Could you check a few things on this model? Use its own coordinates, in mm. A direction names the side the tool comes from. Give positions to 0.01 mm unless a question says otherwise; leave off trailing zeros. Loops run counter-clockwise (first coordinate to the right, second up) from the corner with the lowest first, then second, coordinate; pieces in that order, holes last. Notation, with made-up numbers: (-34, 17.25) - (-3, 17.25) arc R25 cw to (-3, 48.25) - close; hole circle Ø11 at (-37, -16). An arc over 180 degrees is marked (long way). Write each question's results on one line, items separated by ' | '. Start each with the question number.
(1) Suppose I cut it at A-A (y = 1). Please give me the cut outline in (x, z).
(2) Suppose I cut it at B-B (x = 13.97). Please give me the cut outline in (y, z), and give its area (3 significant figures).
(3) Suppose I cut it at D-D (y = -1.75). Please give me the cut outline in (x, z).
(4) If we mould it in two halves opening along Y, with no side actions, what happens to faces 1 (the face through (15.42, -0.06, 2.03)), 2 (the face through (0, -6.6, 2)), 3 (the face through (-16.7, 0, 2))? For each: released by +Y, released by -Y, zero draft, split by the parting line, or undercut.
(5) Suppose I cut it at C-C (z = 0.8). Please give me the cut outline in (x, y).
(6) For pin 1 (4.5 mm diameter, centred on x = 13.97, y = 0, fed in from -Z), with a flat end and sliding along its axis, tell me the tip position at first contact or that it passes through.
(7) I need wall thicknesses on line 1 (X direction, y = 1.5, z = 1.3); line 2 (Y direction, x = 5.5, z = 2.1); line 3 (Y direction, x = -13.97, z = 1.9). Which ranges of each line are inside material? Lowest first, please.
(8) On a 3-axis mill with a long thin cutter (end or side, diameter ignored), from which of +Z, -Z, +X, -X, +Y, -Y can I reach the whole of each face in a straight line? I mean faces 4 (the face through (0, 6.6, 2)), 5 (the face through (0, 6, 2)). Say none if no direction works.
from build123d import *

# Parameters (mm, degrees)
SKETCH1_W            = 33.4
SKETCH1_H            = 13.2
SKETCH1_W_2          = 32.2
SKETCH1_H_2          = 12
BOSS_EXTRUDE3_DEPTH  = 4
SKETCH3_W            = 4.9276
SKETCH3_H            = 12
BOSS_EXTRUDE4_DEPTH  = 4
SKETCH4_R            = 1.45
MOUNTING_HOLES_DEPTH = 19.397010627


with BuildPart() as part:
    # Sketch1 → Boss-Extrude3 (new body)
    with BuildSketch(Plane.XY):
        Rectangle(SKETCH1_W, SKETCH1_H)
        Rectangle(SKETCH1_W_2, SKETCH1_H_2, mode=Mode.SUBTRACT)
    extrude(amount=BOSS_EXTRUDE3_DEPTH)

    # Sketch3 → Boss-Extrude4 (add, through all)
    with BuildSketch(Plane.XY.offset(4)):
        with Locations((-13.6362, 0)):
            Rectangle(SKETCH3_W, SKETCH3_H)
        with Locations((13.6362, 0)):
            Rectangle(SKETCH3_W, SKETCH3_H)
    extrude(amount=-BOSS_EXTRUDE4_DEPTH)

    # Sketch4 → mounting holes (cut, through all)
    with BuildSketch(Plane.XY.offset(4)):
        with Locations((-13.97, 0)):
            Circle(SKETCH4_R)
        with Locations(Location((13.97, 0, 0), (0, 0, 180))):
            Circle(SKETCH4_R)
    extrude(amount=-MOUNTING_HOLES_DEPTH, mode=Mode.SUBTRACT)


solid = part.part
Output values:
1) outline: (-16.7, 0) - (-15.02, 0) - (-15.02, 4) - (-16.7, 4) - close; (-12.92, 0) - (-11.17, 0) - (-11.17, 4) - (-12.92, 4) - close; (11.17, 0) - (12.92, 0) - (12.92, 4) - (11.17, 4) - close; (15.02, 0) - (16.7, 0) - (16.7, 4) - (15.02, 4) - close
2) outline: (-6.6, 0) - (-1.45, 0) - (-1.45, 4) - (-6.6, 4) - close; (1.45, 0) - (6.6, 0) - (6.6, 4) - (1.45, 4) - close | area: 41.2 mm2
3) outline: (-16.7, 0) - (-11.17, 0) - (-11.17, 4) - (-16.7, 4) - close; (11.17, 0) - (16.7, 0) - (16.7, 4) - (11.17, 4) - close
4) face 1: undercut | face 2: released by -Y | face 3: zero draft
5) outline: (-16.7, -6.6) - (16.7, -6.6) - (16.7, 6.6) - (-16.7, 6.6) - close; hole circle Ø2.9 at (-13.97, 0); hole (-11.17, -6) - (11.17, -6) - (11.17, 6) - (-11.17, 6) - close; hole circle Ø2.9 at (13.97, 0)
6) pin 1: z = 0
7) line 1: -16.7 to -11.17, 11.17 to 16.7 | line 2: -6.6 to -6, 6 to 6.6 | line 3: -6.6 to -1.45, 1.45 to 6.6
8) face 4: +Z, -Z, +X, -X, +Y | face 5: +Z, -Z
